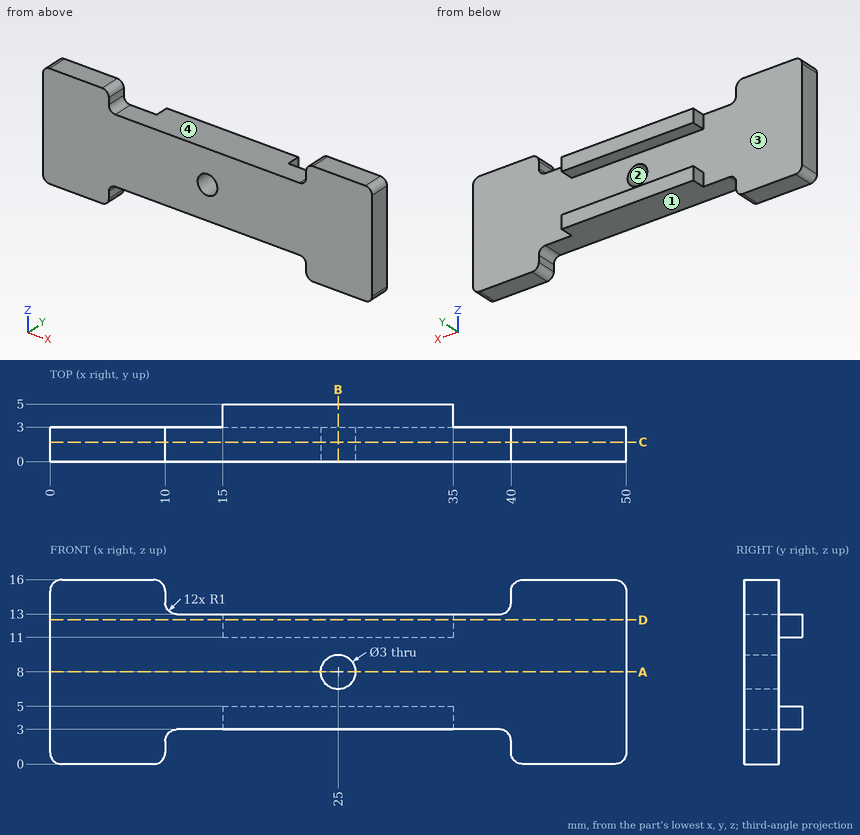
Geometry: see drawing. Coordinates: mm, zero at the bounding-box minimum. A direction names the side the tool comes from. Give positions to 0.01 mm unless a question says otherwise; leave off trailing zeros. Write each loop counter-clockwise with the first axis right and the second up, starting at its lowest first coordinate (ties: lowest second). Pieces come first, ordered by that corner, then holes. Notation, with made-up numbers: (-23.75, -0.75) - (30.25, -0.75) arc R16 cw to (30.25, 6.25) - close; hole circle Ø3 at (77.5, -29). An arc over 180 degrees is marked (long way). Return JSON: item names as keys, results as strings. Group by question number.
1) Section A-A on z = 8. Return the cut outline in (x, y).
2) Section B-B on x = 25. Return the cut outline in (y, z).
3) Section D-D on z = 12.5. Return the cut outline in (x, y).
4) Line query: line 1 (X direction, y = 0.9, z = 8); line 2 (Z direction, x = 28, y = 4); line 3 (X direction, y = 2.1, z = 1.25). Output: solid intervals per line, ascending.
5) Set-up query: the marked faces 1 and 2. Return all of +Z, -Z, +X, -X, +Y, -Y with unobstructed straight access to the full face (end or side cutting, diameter ignored); none if empty.
6) Section C-C on y = 1.7. Return the cut outline in (x, z).
7) Mould query, pull axis X, two halves, no side actions, for the marked faces 3 and 4. Classes: released by +X, released by -X, zero draft, split by the parting line, or undercut.
8) First-contact query: P1, Ø0.6, axis at y = 4, z = 12, coming from the +X side; P2, Ø0.6, axis at y = 4.5, z = 12, coming from the -X side; P3, Ø0.6, axis at x = 26.5, y = 4, coming from the +Z side. Flat tips, straight axial feed; report the tip coordinate or a pass-through.
Filled in:
{
 "1": {"outline": "(0, 0) - (23.5, 0) - (23.5, 3) - (0, 3) - close; (26.5, 0) - (50, 0) - (50, 3) - (26.5, 3) - close"},
 "2": {"outline": "(0, 3) - (5, 3) - (5, 5) - (3, 5) - (3, 6.5) - (0, 6.5) - close; (0, 9.5) - (3, 9.5) - (3, 11) - (5, 11) - (5, 13) - (0, 13) - close"},
 "3": {"outline": "(0, 0) - (50, 0) - (50, 3) - (35, 3) - (35, 5) - (15, 5) - (15, 3) - (0, 3) - close"},
 "4": {"line 1": "x = 0 to 23.5, 26.5 to 50", "line 2": "z = 3 to 5, 11 to 13", "line 3": "x = 0 to 10, 40 to 50"},
 "5": {"face 1": "-Z, +Y, -Y", "face 2": "+Y, -Y"},
 "6": {"outline": "(0, 1) arc R1 ccw to (1, 0) - (9, 0) arc R1 ccw to (10, 1) - (10, 2) arc R1 cw to (11, 3) - (39, 3) arc R1 cw to (40, 2) - (40, 1) arc R1 ccw to (41, 0) - (49, 0) arc R1 ccw to (50, 1) - (50, 15) arc R1 ccw to (49, 16) - (41, 16) arc R1 ccw to (40, 15) - (40, 14) arc R1 cw to (39, 13) - (11, 13) arc R1 cw to (10, 14) - (10, 15) arc R1 ccw to (9, 16) - (1, 16) arc R1 ccw to (0, 15) - close; hole circle Ø3 at (25, 8)"},
 "7": {"face 3": "zero draft", "face 4": "undercut"},
 "8": {"P1": "stops at x = 35", "P2": "stops at x = 15", "P3": "stops at z = 13"}
}
